from build123d import *

# Parameters (mm, degrees)
SKETCH1_W             = 368.3
SKETCH1_H             = 228.6
BOSS_EXTRUDE1_DEPTH   = 4.7625
CUT_EXTRUDE1_DEPTH    = 217.791129676
SKETCH_PATTERN1_DEPTH = 4.7625
FILLET1_R             = 2.54
F_8_CLEARANCE_HOLE1_D = 4.3053


# Read off the part's stored shape, not the designer's step: Sketch-Pattern1
with BuildPart() as part:
    # Sketch1 → Boss-Extrude1 (new body)
    with BuildSketch(Plane(origin=(0, 0, 0), x_dir=(1, 0, 0), z_dir=(0, 1, 0))):
        Rectangle(SKETCH1_W, SKETCH1_H)
    extrude(amount=BOSS_EXTRUDE1_DEPTH)

    # Sketch3 → Cut-Extrude1 (cut, through all)
    with BuildSketch(Plane.XZ):
        with BuildLine():
            Line((143.533374481, -3.245454654), (95.226625519, -3.245454654))
            ThreePointArc((95.226625519, -3.245454654), (63.594954654, -53.5305), (95.226625519, -103.815545346))
            Line((95.226625519, -103.815545346), (143.533374481, -103.815545346))
            ThreePointArc((143.533374481, -103.815545346), (175.165045346, -53.5305), (143.533374481, -3.245454654))
        make_face()
    extrude(amount=-CUT_EXTRUDE1_DEPTH, mode=Mode.SUBTRACT)

    # Sketch-Pattern1 outline → Sketch-Pattern1 (cut)
    with BuildSketch(Plane(origin=(0, 0, 0), x_dir=(1, 0, 0), z_dir=(0, 1, 0))):
        with BuildLine():
            ThreePointArc((-24.153374481, 103.815545346), (-55.785045346, 53.5305), (-24.153374481, 3.245454654))
            Line((-24.153374481, 3.245454654), (24.153374481, 3.245454654))
            ThreePointArc((24.153374481, 3.245454654), (55.785045346, 53.5305), (24.153374481, 103.815545346))
            Line((24.153374481, 103.815545346), (-24.153374481, 103.815545346))
        make_face()
        with BuildLine():
            ThreePointArc((-143.533374481, 103.815545346), (-175.165045346, 53.5305), (-143.533374481, 3.245454654))
            Line((-143.533374481, 3.245454654), (-95.226625519, 3.245454654))
            ThreePointArc((-95.226625519, 3.245454654), (-63.594954654, 53.5305), (-95.226625519, 103.815545346))
            Line((-95.226625519, 103.815545346), (-143.533374481, 103.815545346))
        make_face()
        with BuildLine():
            ThreePointArc((95.226625519, -3.245454654), (63.594954654, -53.5305), (95.226625519, -103.815545346))
            Line((95.226625519, -103.815545346), (143.533374481, -103.815545346))
            ThreePointArc((143.533374481, -103.815545346), (175.165045346, -53.5305), (143.533374481, -3.245454654))
            Line((143.533374481, -3.245454654), (95.226625519, -3.245454654))
        make_face()
        with BuildLine():
            ThreePointArc((-24.153374481, -3.245454654), (-55.785045346, -53.5305), (-24.153374481, -103.815545346))
            Line((-24.153374481, -103.815545346), (24.153374481, -103.815545346))
            ThreePointArc((24.153374481, -103.815545346), (55.785045346, -53.5305), (24.153374481, -3.245454654))
            Line((24.153374481, -3.245454654), (-24.153374481, -3.245454654))
        make_face()
        with BuildLine():
            ThreePointArc((-143.533374481, -3.245454654), (-175.165045346, -53.5305), (-143.533374481, -103.815545346))
            Line((-143.533374481, -103.815545346), (-95.226625519, -103.815545346))
            ThreePointArc((-95.226625519, -103.815545346), (-63.594954654, -53.5305), (-95.226625519, -3.245454654))
            Line((-95.226625519, -3.245454654), (-143.533374481, -3.245454654))
        make_face()
    extrude(amount=SKETCH_PATTERN1_DEPTH, mode=Mode.SUBTRACT)

    # Fillet1
    fillet1_edges = [part.edges().sort_by_distance(p)[0] for p in [
        (184.15, 2.38125, 114.3),
        (-184.15, 2.38125, 114.3),
        (-184.15, 2.38125, -114.3),
        (184.15, 2.38125, -114.3),
    ]]
    fillet(fillet1_edges, radius=FILLET1_R)

    # #8 Clearance Hole1 (through all)
    with Locations(Plane(origin=(0, 0, 0), x_dir=(-1, 0, 0), z_dir=(0, -1, 0))):
        with Locations((-178.907772673, 109.057772673), (-59.69, 109.057772673), (59.69, 109.057772673), (178.907772673, 109.057772673), (178.907772673, -109.057772673), (59.69, -109.057772673), (-59.69, -109.057772673), (-178.907772673, -109.057772673), (59.69, 0), (-59.69, 0)):
            Hole(F_8_CLEARANCE_HOLE1_D / 2)


solid = part.part
Could you check a few things on this model? Use its own coordinates, in mm. A direction names the side the tool comes from. Give positions to 0.01 mm unless a question says otherwise; leave off trailing zeros. Write each loop counter-clockwise with the first axis right and the second up, starting at its lowest first coordinate (ties: lowest second). Pieces come first, ordered by that corner, then holes. Notation, with made-up numbers: (-3, 69.5) -> (4, 69.5) arc R9 cw to (4, 77.5) -> close; hole circle Ø4 at (17.25, -1). An arc over 180 degrees is marked (long way). Answer as a JSON object with one key per item and string values.
Q1. Please list where these lines run through material, in increasing order: L1, parallel to Z at x = 59.69, y = 3.35; L2, parallel to Z at x = 116.5, y = 1.25; L3, parallel to X at y = 3.15, z = -4.5.
Taken from the geometry:
{"L1": "z = -114.3 to -111.21, -106.91 to -2.15, 2.15 to 106.91, 111.21 to 114.3", "L2": "z = -114.3 to -103.82, -3.25 to 3.25, 103.82 to 114.3", "L3": "x = -184.15 to -145.99, -92.77 to -26.61, 26.61 to 92.77, 145.99 to 184.15"}
Q2. We'd pull the mould along Z, two halves only. Please class faces 3 (the cylindrical face through (55.78, 2.35, 54.41)), 4 (the flat face through (-1, 4.762, -1)): released by +Z, released by -Z, zero draft, split by the parting line, or undercut.
Taken from the geometry:
{"face 3": "undercut", "face 4": "zero draft"}
Q3. Suppose I cut it at A-A on x = -3. Write out the boundary of the cut face in (y, z), then the cut area to 3 significant figures.
Taken from the geometry:
{"outline": "(0, -114.3) -> (4.76, -114.3) -> (4.76, -103.82) -> (0, -103.82) -> close; (0, -3.25) -> (4.76, -3.25) -> (4.76, 3.25) -> (0, 3.25) -> close; (0, 103.82) -> (4.76, 103.82) -> (4.76, 114.3) -> (0, 114.3) -> close", "area": "131 mm²"}
Q4. Suppose I cut it at C-C on z = 58. Write out the boundary of the cut face in (x, y), then the cut area to 3 significant figures.
Taken from the geometry:
{"outline": "(-184.15, 0) -> (-174.99, 0) -> (-174.99, 4.76) -> (-184.15, 4.76) -> close; (-63.77, 0) -> (-55.61, 0) -> (-55.61, 4.76) -> (-63.77, 4.76) -> close; (55.61, 0) -> (63.77, 0) -> (63.77, 4.76) -> (55.61, 4.76) -> close; (174.99, 0) -> (184.15, 0) -> (184.15, 4.76) -> (174.99, 4.76) -> close", "area": "165 mm²"}
Q5. Which directions (+Z, -Z, +X, -X, +Y, -Y) give clear straight access to the entire face, cutting with the end or side of a thin tool? Please do faces 1 (the flat face through (-1, 0, -1)), 2 (the cylindrical face through (175.16, 2.35, -54.41)).
Taken from the geometry:
{"face 1": "+Z, -Z, +X, -X, -Y", "face 2": "+Y, -Y"}
Q6. Suppose I cut it at B-B on z = -56.5. Write out the boundary of the cut face in (x, y), then the cut area to 3 significant figures.
Taken from the geometry:
{"outline": "(-184.15, 0) -> (-175.09, 0) -> (-175.09, 4.76) -> (-184.15, 4.76) -> close; (-63.67, 0) -> (-55.71, 0) -> (-55.71, 4.76) -> (-63.67, 4.76) -> close; (55.71, 0) -> (63.67, 0) -> (63.67, 4.76) -> (55.71, 4.76) -> close; (175.09, 0) -> (184.15, 0) -> (184.15, 4.76) -> (175.09, 4.76) -> close", "area": "162 mm²"}
Q7. Suppose I cut it at D-D on y = 0.85. Count the separate pieces of the cut face and the enclosed holes in it, then the cut area to 3 significant figures.
Taken from the geometry:
{"separate pieces": "1", "enclosed holes": "16", "area": "27,500 mm²"}
